Job drawing, mm, ordinate dimensions from the low corner. One solid piece. A direction names the side the tool comes from. Round coordinates to 2 decimals unless told otherwise and drop trailing zeros. Loops run counter-clockwise (first coordinate to the right, second up) from the corner with the lowest first, then second, coordinate; pieces in that order, holes last. Notation, with made-up numbers: M 48,40 L 53,40 A34 ccw 53,71 Z; hole C 3,-11.75 d10. An arc over 180 degrees is marked long. Use one line per item in the form item = value. Start each with the question number.
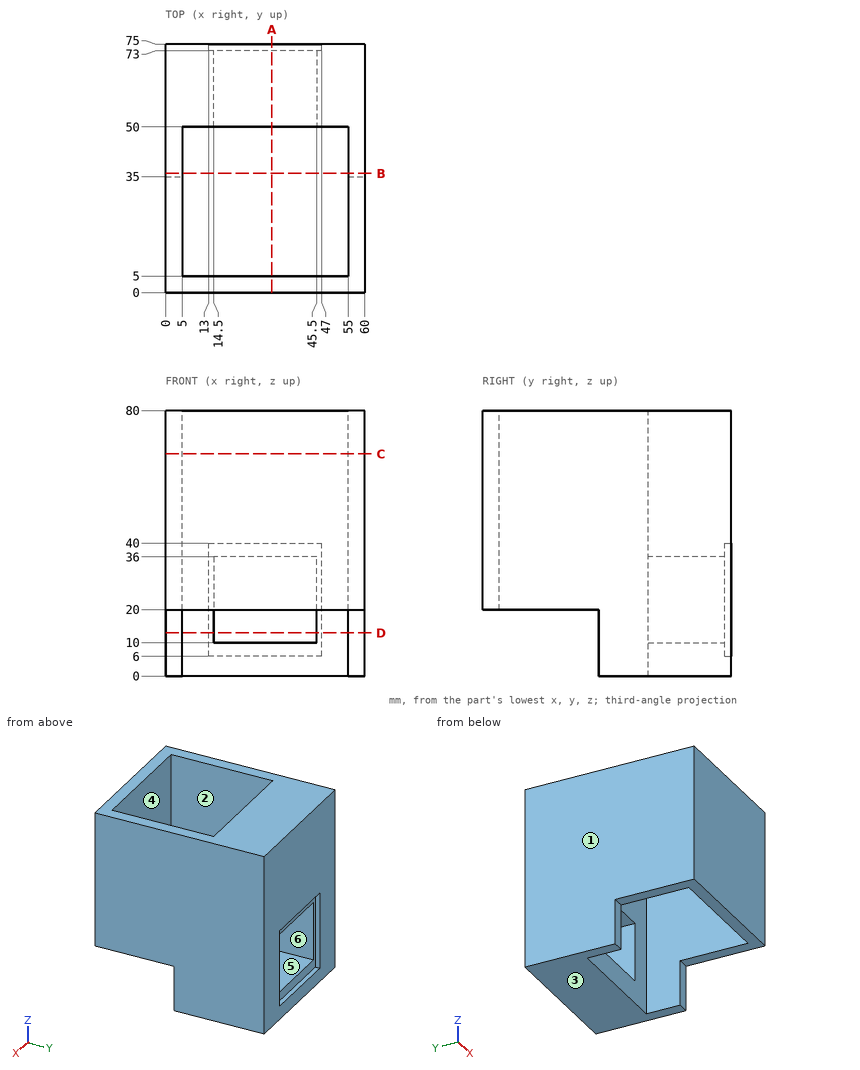
Q1. Saw through at B-B (y = 36). Give the cut face in (x, z).
Q2. Saw through at C-C (z = 67). Give the cut face in (x, y), and give its area (3 significant figures).
Q3. Saw through at A-A (x = 32). Give the cut face in (y, z).
Q4. Saw through at D-D (z = 13). Give the cut face in (x, y), and give its area (3 significant figures).
Q5. Drop flat-ended pins along their axis: P1, Ø2, axis at y = 34.5, z = 56.5, coming from the -X side; P2, Ø10, axis at x = 38, z = 22, coming from the +Y side; P3, Ø4, axis at x = 2.5, z = 9, coming from the -Y side; P4, Ø12, axis at x = 16, z = 13.5, coming from the -Y side. Give the stop position or say it passes through.
Q6. Tool access for the marked faces 4, 5 and 6: list every direction of +Z, -Z, +X, -X, +Y, -Y with a clear straight run to the whole face (end or side of a thin tool).
Q7. Pull direction X, two halves, no side cores. Call the marked faces 1, 2 and 3: pulls with the +X half, pulls with the -X half, needs draft (parallel to the pull), parting line crosses it, or undercut.
Q8. Wall check: probe 1 along X at (y, z) = (17.5, 62); probe 2 along Y at (x, z) = (14, 65); probe 3 along X at (y, z) = (64.5, 25.5). Give the ranges that are in metal, low to high.
Filled in:
q1.outline = M 0,0 L 5,0 L 5,80 L 0,80 Z; M 55,0 L 60,0 L 60,80 L 55,80 Z
q2.outline = M 0,0 L 60,0 L 60,75 L 0,75 Z; hole M 5,5 L 55,5 L 55,50 L 5,50 Z
q2.area = 2,250 mm²
q3.outline = M 0,20 L 5,20 L 5,80 L 0,80 Z; M 50,0 L 75,0 L 75,6 L 73,6 L 73,10 L 50,10 Z; M 50,36 L 73,36 L 73,40 L 75,40 L 75,80 L 50,80 Z
q4.outline = M 0,35 L 5,35 L 5,50 L 14.5,50 L 14.5,73 L 13,73 L 13,75 L 0,75 Z; M 45.5,50 L 55,50 L 55,35 L 60,35 L 60,75 L 47,75 L 47,73 L 45.5,73 Z
q4.area = 869 mm²
q5.P1 = 0
q5.P2 = 5
q5.P3 = 35
q5.P4 = 50
q6.face_4 = +Z, -Z
q6.face_5 = +Y, -Y
q6.face_6 = +Y
q7.face_1 = pulls with the -X half
q7.face_2 = undercut
q7.face_3 = needs draft
q8.probe_1 = 0 to 5, 55 to 60
q8.probe_2 = 0 to 5, 50 to 75
q8.probe_3 = 0 to 14.5, 45.5 to 60
